Work out the finished part from the listing and answer in its coordinate system (mm). A direction names the side the tool comes from. Give positions to 0.01 mm unless a question says otherwise; leave off trailing zeros. Order: outer loops, then holes, each group sorted by start corner. A loop starts at its lowest first (then second) coordinate and runs counter-clockwise, first axis right, second up. Notation, with made-up numbers: M -3,40 L 36,40 A16 ccw 36,67 Z; hole C -26,2 d7. An arc over 180 degrees is marked long. One line per item, written item: value.
from build123d import *

# Parameters (mm, degrees)
BOSS_EXTRUDE1_DEPTH = 1.5875


with BuildPart() as part:
    # Sketch2 → Boss-Extrude1 (new, symmetric)
    with BuildSketch(Plane.XY):
        with BuildLine():
            Line((55.130521201, -12.193939448), (51.93209544, 1.905344025))
            ThreePointArc((51.93209544, 1.905344025), (49.621085039, 5.5280528), (45.533364229, 6.85294016))
            ThreePointArc((45.533364229, 6.85294016), (41.466923822, 5.464109588), (39.213011171, 1.80560365))
            Line((39.213011171, 1.80560365), (36.236092368, -12.342105573))
            Line((36.236092368, -12.342105573), (39.283717526, -12.294304966))
            ThreePointArc((39.283717526, -12.294304966), (41.213777682, -16.754713179), (45.732521201, -18.543939448))
            ThreePointArc((45.732521201, -18.543939448), (50.222649262, -16.684067509), (52.082521201, -12.193939448))
            Line((52.082521201, -12.193939448), (55.130521201, -12.193939448))
        make_face()
    extrude(amount=BOSS_EXTRUDE1_DEPTH, both=True)


solid = part.part
(1) Given P1, Ø1.5, axis at y = -15, z = 1, coming from the -X side, flat-ended and moving along its own axis, determine where the tip first touches the part or whether it passes through.
Findings:
P1: stops at x = 39.62
(2) Find the intervals of material crossed by probe 1 along X at (y, z) = (-17.5, -1.2); probe 2 along Y at (x, z) = (41.5, -0.45); probe 3 along Y at (x, z) = (47.5, -1), in increasing order. Write a range as from..to.
Findings:
probe 1: x = 42.14..49.22
probe 2: y = -17.02..5.49
probe 3: y = -18.29..6.61
(3) Section C-C, the plane y = -2.25 is taken. Give the vertices of the cut face in (x, z).
Findings:
outline: M 38.36,-1.59 L 52.87,-1.59 L 52.87,1.59 L 38.36,1.59 Z
(4) Section B-B, the plane x = 42 is taken. Give the vertices of the cut face in (y, z), then the cut area to 3 significant figures.
Findings:
outline: M -17.4,-1.59 L 5.85,-1.59 L 5.85,1.59 L -17.4,1.59 Z
area: 73.8 mm^2
(5) Which of the six approach directions +Z, -Z, +X, -X, +Y, -Y give full straight-line access (tool end or side, diameter ignored) to faces 1 (the flat face through (54, -12.194, 0)), 2 (the flat face through (46, -6, -1.588))?
Findings:
face 1: +Z, -Z, +X, -Y
face 2: -Z, +X, -X, +Y, -Y
(6) Section A-A, the plane z = 0.3 is taken. Give the vertices of the cut face in (x, y), then the cut area to 3 significant figures.
Findings:
outline: M 36.24,-12.34 L 39.28,-12.29 A6.35 ccw 45.73,-18.54 A6.35 ccw 52.08,-12.19 L 55.13,-12.19 L 51.93,1.91 A6.36 ccw 45.53,6.85 A6.36 ccw 39.21,1.81 Z
area: 334 mm^2
